from build123d import *

# Parameters (mm, degrees)
SKETCH_W        = 9.9
SKETCH_H        = 58
PAD_DEPTH       = 40
SKETCH001_W     = 9.9
SKETCH001_H     = 43
POCKET_DEPTH    = 30
FILLET_R        = 29.9
SKETCH002_R     = 3
POCKET001_DEPTH = 34
SKETCH003_R     = 1.9
POCKET002_DEPTH = 6


with BuildPart() as part:
    # Sketch → Pad (new body)
    with BuildSketch(Plane.XY):
        Rectangle(SKETCH_W, SKETCH_H)
    extrude(amount=PAD_DEPTH)

    # Sketch001 (on Face6 of Pad) → Pocket (cut)
    with BuildSketch(Plane.XY.offset(40)):
        with Locations((0, -7.5)):
            Rectangle(SKETCH001_W, SKETCH001_H)
    extrude(amount=-POCKET_DEPTH, mode=Mode.SUBTRACT)

    # Fillet
    fillet_edges = [part.edges().sort_by_distance(p)[0] for p in [
        (0, 14, 10),
    ]]
    fillet(fillet_edges, radius=FILLET_R)

    # Sketch002 (on Face4 of Fillet) → Pocket001 (cut)
    with BuildSketch(Plane.XY.offset(40)):
        with Locations((0, 9)):
            Circle(SKETCH002_R)
        with Locations((0, -11)):
            Circle(SKETCH002_R)
    extrude(amount=-POCKET001_DEPTH, mode=Mode.SUBTRACT)

    # Sketch003 (on Face8 of Pocket001) → Pocket002 (cut)
    with BuildSketch(Plane(origin=(0, 0, 0), x_dir=(1, 0, 0), z_dir=(0, 0, -1))):
        with Locations((0, -9)):
            Circle(SKETCH003_R)
        with Locations((0, 11)):
            Circle(SKETCH003_R)
    extrude(amount=-POCKET002_DEPTH, mode=Mode.SUBTRACT)


solid = part.part
Work out the finished part from the listing and answer in its coordinate system (mm). A direction names the side the tool comes from. Round coordinates to 2 decimals unless told otherwise and drop trailing zeros. Loops run counter-clockwise (first coordinate to the right, second up) from the corner with the lowest first, then second, coordinate; pieces in that order, holes last. Notation, with made-up numbers: (79, -21.75) - (109, -21.75) arc R10 cw to (109, -8.75) - close; hole circle Ø9 at (51, 31). An arc over 180 degrees is marked (long way). One line per item, written item: value.
Q1. Each of these flat-tipped pins is pushed along its axis until it touches: pin 1 Ø1 at (x, z) = (-2.5, 20) entering from -Y; pin 2 Ø3 at (x, y) = (0, -11) entering from -Z; pin 3 Ø1.8 at (x, y) = (1, 9.5) entering from +Z. Where does it stop, or does it pass through?
Check values:
pin 1: y = 5.96
pin 2: through
pin 3: z = 6
Q2. Straight lines are drawn through the part: probe 1 along Y at (x, z) = (0, 3.85); probe 2 along Y at (x, z) = (-2.25, 6.5); probe 3 along X at (y, z) = (9, 1). For each, find the intervals that lie inside material, in ascending order.
Check values:
probe 1: -29 to -12.9, -9.1 to 7.1, 10.9 to 29
probe 2: -29 to -12.98, -9.02 to 7.02, 10.98 to 29
probe 3: -4.95 to -1.9, 1.9 to 4.95
Q3. Find section A-A on y = -11. Give the vertices of the cut face in (x, z).
Check values:
outline: (-4.95, 0) - (-1.9, 0) - (-1.9, 6) - (-3, 6) - (-3, 10.4) - (-4.95, 10.4) - close; (1.9, 0) - (4.95, 0) - (4.95, 10.4) - (3, 10.4) - (3, 6) - (1.9, 6) - close
Q4. For faces 1 (the cylindrical face through (0.877, 10.686, 2.958)), 2 (the flat face through (0, -22, 10)), 3 (the cylindrical face through (0, -8, 8)), determine the directions among +Z, -Z, +X, -X, +Y, -Y from which every point of the face is accessible in a straight line to the end or side of a thin tool.
Check values:
face 1: +Z, -Z
face 2: +Z, +X, -X, -Y
face 3: +Z
Q5. The mould has two halves that part along X. Classify faces 4 (the flat face through (1, 7, 6)), 5 (the cylindrical face through (0, 12, 15)), 6 (the flat face through (0, 29, 20)), 7 (the flat face through (-4.95, 6, 15)): +X half, -X half, draft (parallel to the pull), parting line (faces both ways), or undercut.
Check values:
face 4: undercut
face 5: undercut
face 6: draft
face 7: -X half
Q6. Find section D-D on y = -17. Give the vertices of the cut face in (x, z), and give its area (3 significant figures).
Check values:
outline: (-4.95, 0) - (4.95, 0) - (4.95, 10) - (-4.95, 10) - close
area: 99.0 mm2
Q7. Find section B-B on x = -0.25. Give the vertices of the cut face in (y, z).
Check values:
outline: (-29, 0) - (-12.88, 0) - (-12.88, 6) - (-13.99, 6) - (-13.99, 10.06) arc R29.9 cw to (-15.9, 10) - (-29, 10) - close; (-9.12, 0) - (7.12, 0) - (7.12, 6) - (6.01, 6) - (6.01, 19.55) arc R29.9 cw to (-8.01, 11.06) - (-8.01, 6) - (-9.12, 6) - close; (10.88, 0) - (29, 0) - (29, 40) - (14, 40) - (14, 39.9) arc R29.9 cw to (11.99, 29.12) - (11.99, 6) - (10.88, 6) - close
Q8. Find section C-C on z = 22.5. Give the vertices of the cut face in (x, y).
Check values:
outline: (-4.95, 8.42) - (-2.94, 8.42) arc R3 cw (long way) to (2.94, 8.42) - (4.95, 8.42) - (4.95, 29) - (-4.95, 29) - close
